Verification items for the finished model (mm, model axes). Give positions to 0.01 mm unless a question says otherwise; leave off trailing zeros. Order: outer loops, then holes, each group sorted by start corner. A loop starts at its lowest first (then second) coordinate and runs counter-clockwise, first axis right, second up. Notation, with made-up numbers: M 78,-2.5 L 130,-2.5 A30 cw 130,30.5 Z; hole C 67.25,32.25 d1. An arc over 180 degrees is marked long. Answer as a JSON object with one key per item and string values.
Autodesk Inventor part; units mm, degrees
ref_plane "Work Plane2" through (19.05, -1.5, 88.9) normal (-0.7071, -0.7071, 0) x (0, 0, 1)
ref_plane "YZ Plane" through (0, 0, 0) normal (1, 0, 0) x (0, 1, 0)
ref_plane "XZ Plane" through (0, 0, 0) normal (0, 1, 0) x (-1, 0, 0)
sketch "Sketch1" plane through (0, 0, 0) normal (0, 1, 0) x (-1, 0, 0)
  line L0 (-19.05, 49.2125) -> (19.05, 49.2125)
  line L1 (19.05, 49.2125) -> (19.05, -49.2125)
  line L2 (19.05, -49.2125) -> (-19.05, -49.2125)
  line L3 (-19.05, -49.2125) -> (-19.05, 49.2125)
  line L4 (-19.05, 49.2125) -> (19.05, -49.2125) construction
  line L5 (19.05, 49.2125) -> (-19.05, -49.2125) construction
  line L6 (19.05, 0) -> (-19.05, 0) construction
  line L7 (-19.05, -49.2125) -> (19.05, -49.2125) construction
  line L8 (19.05, -49.2125) -> (19.05, -87.3125)
  line L9 (19.05, -87.3125) -> (-19.05, -87.3125)
  line L10 (-19.05, -87.3125) -> (-19.05, -49.2125)
  line L11 (19.05, -49.2125) -> (-19.05, -63.0798)
  line L12 (19.05, 49.2125) -> (-19.05, 49.2125) construction
  line L13 (-19.05, 49.2125) -> (19.05, 49.2125) construction
  line L14 (19.05, 49.2125) -> (19.05, 87.3125)
  line L15 (19.05, 87.3125) -> (-19.05, 87.3125)
  line L16 (-19.05, 87.3125) -> (-19.05, 49.2125)
  line L17 (19.05, 49.2125) -> (-19.05, 63.0798)
  line L18 (19.05, 42.8625) -> (-19.05, 42.8625) construction
  line L19 (-19.05, -63.0798) -> (9.525, -87.3125)
  line L20 (-19.05, 63.0798) -> (9.525, 87.3125)
  point P0 (0, 0)
  point P1 (12.7, 42.8625)
  point P2 (3.175, 42.8625)
  point P3 (-6.35, 42.8625)
  point P4 (12.7, 33.3375)
  point P5 (3.175, 33.3375)
  point P6 (-6.35, 33.3375)
  point P7 (12.7, -42.8625)
  point P8 (3.175, -42.8625)
  point P9 (-6.35, -42.8625)
  point P10 (12.7, -33.3375)
  point P11 (3.175, -33.3375)
  point P12 (-6.35, -33.3375)
  point P13 (19.05, 49.2125)
  point P14 (9.525, 87.3125)
  point P15 (19.05, 49.2125)
  point P16 (-19.05, 63.0798)
  dimension "d0" = 38.1
  dimension "d1" = 98.425
  dimension "d2" = 38.1
  dimension "d3" = 38.1
  dimension "d5" = 20
  dimension "d20" = 6.35
  dimension "d23" = 9.525
  dimension "d26" = 9.525
  dimension "d29" = 6.35
  dimension "d33" = 28.575
extrude "Extrusion1" add sketch "Sketch1" against normal blind 1.5875 contours L16 L17 L0 | L0 L1 L2 L3 | L2 L11 L10
ref_plane "Work Plane2" through (19.05, -1.5, 88.9) normal (-0.7071, -0.7071, 0) x (0, 0, 1)
feature "Bend Part3" [suppressed]
feature "Bend Part4" [suppressed]
sketch "Sketch2" plane through (19.05, -1.5, 88.9) normal (-0.7071, -0.7071, 0) x (0, 0, 1)
  line L0 (-10.6966, 1.0607) -> (-167.1034, 1.0607)
  line L1 (-167.1034, 1.0607) -> (-167.1034, -24.3393)
  line L2 (-167.1034, -24.3393) -> (-10.6966, -24.3393)
  line L3 (-10.6966, -24.3393) -> (-10.6966, 1.0607)
  line L4 (-10.6966, 1.0607) -> (-167.1034, 1.0607)
  line L5 (-167.1034, 1.0607) -> (-167.1034, 3.4419)
  line L6 (-167.1034, 3.4419) -> (-10.6966, 3.4419)
  line L7 (-10.6966, 3.4419) -> (-10.6966, 1.0607)
  point P0 (-88.9, 14.531)
  point P1 (-153.5673, 1.0607)
  point P2 (-167.1034, -7.4895)
  point P3 (-10.6966, -7.4895)
  dimension "d31" = 25.4
  dimension "d32" = 2.3813
extrude "Extrusion2" cut sketch "Sketch2" along normal through all both and the other way through all
hole "Hole1" at (-12.7, 0, 42.8625) at (-3.175, 0, 42.8625) at (6.35, 0, 42.8625) at (-12.7, 0, 33.3375) at (-3.175, 0, 33.3375) at (6.35, 0, 33.3375) at (6.35, 0, -33.3375) at (-3.175, 0, -33.3375) at (-12.7, 0, -33.3375) at (6.35, 0, -42.8625) at (-3.175, 0, -42.8625) at (-12.7, 0, -42.8625) direction (0, -1, 0) diameter 3.2766 end through all countersink diameter 5.715 countersink angle 82
equation "\"d0\" = d2"
properties part number "Wedge" material "Aluminum 6061"
Q1. Section check A-A on y = -0.25. Count the separate pieces of the cut face and the enclosed holes in it, then the cut area to 3 significant figures.
Resolved:
{"separate pieces": "1", "enclosed holes": "12", "area": "3,560 mm²"}
Q2. Release check for a two-part mould opening along X. For faces 1 (the face through (-2, -1.588, 1)), 2 (the face through (-12, -1, -41)), 3 (the face through (-1.927, -0.783, 55.445)) record: +X half, -X half, draft (parallel to the pull), parting line (faces both ways), or undercut.
Resolved:
{"face 1": "draft", "face 2": "undercut", "face 3": "-X half"}
Q3. Gauge pin test, flat ends, axial feed: pin 1 Ø4 at (x, z) = (-12.7, -33.34) entering from +Y; pin 2 Ø4.5 at (x, z) = (-12.7, -42.86) entering from +Y. Record the tip position at first contact, or that the pin passes through.
Resolved:
{"pin 1": "stops at y = -0.98", "pin 2": "stops at y = -0.7"}
Q4. Material ranges on L1, parallel to X at y = -0.4, z = -41; L2, parallel to Z at x = -12.7, y = -1.45; L3, parallel to Z at x = -14, y = -1.1, recorded low to high.
Resolved:
{"L1": "x = -19.05 to -14.38, -11.02 to -4.86, -1.49 to 4.67, 8.03 to 15.28", "L2": "z = -51.52 to -44.5, -41.22 to -34.98, -31.7 to 31.7, 34.98 to 41.22, 44.5 to 51.52", "L3": "z = -51.05 to -44.25, -41.48 to -34.72, -31.95 to 31.95, 34.72 to 41.48, 44.25 to 51.05"}
Q5. Section check C-C on z = 11. Record the cut outline in (x, y).
Resolved:
{"outline": "M -19.05,-1.59 L 14.09,-1.59 L 15.68,0 L -19.05,0 Z"}
